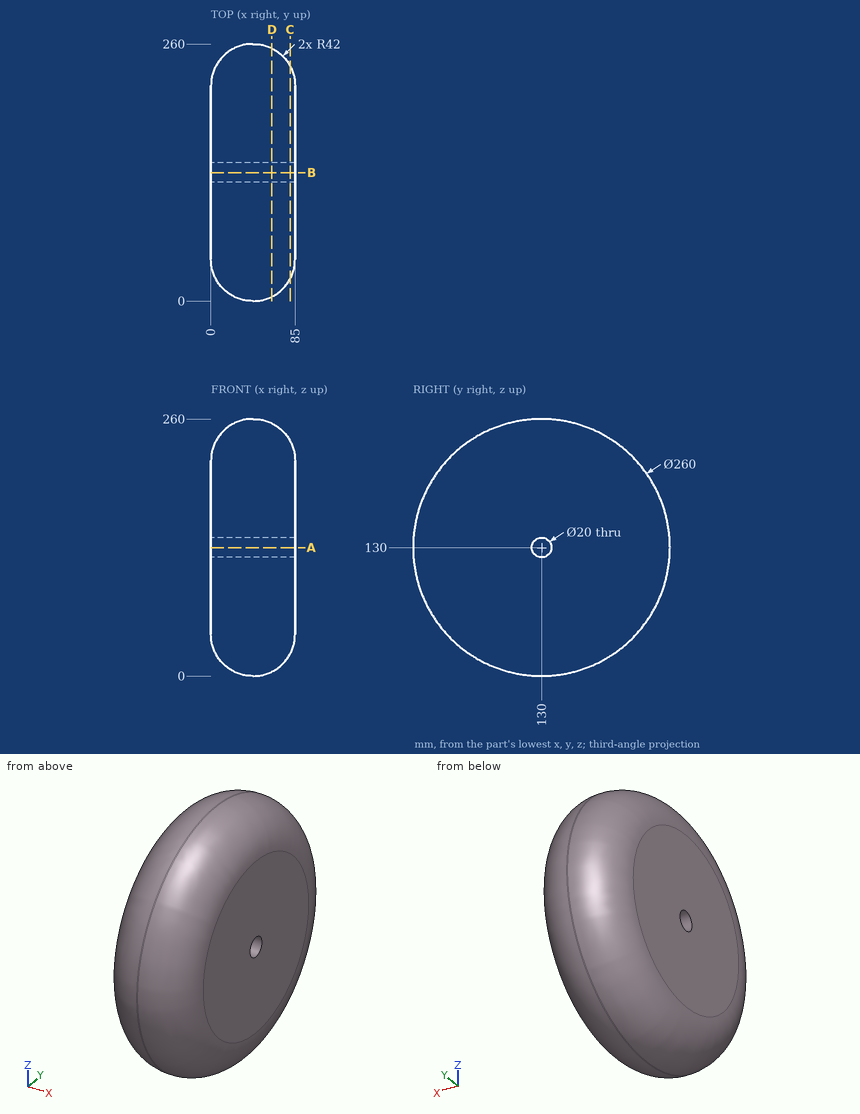
Drawing for the job (mm, zero at the part's lowest x, y, z). Round coordinates to 2 decimals unless told otherwise and drop trailing zeros. Order: outer loops, then holes, each group sorted by start corner. A loop starts at its lowest first (then second) coordinate and runs counter-clockwise, first axis right, second up.
Item 1: Pin check, flat tips, straight feed: pin 1 (8 mm diameter, centred on y = 37.5, z = 58, fed in from +X); pin 2 (5 mm diameter, centred on x = 32, z = 65, fed in from +Y); pin 3 (1.5 mm diameter, centred on x = 33, y = 86, fed in from -Z). Stop position of each tip, or through.
Item 2: Saw through at C-C on x = 80. Write the cut outline in (y, z), then the cut area to 3 significant figures.
Item 3: Probe line 1 along Z through (x, y) = (20, 130); line 2 along Z through (x, y) = (66, 130); line 3 along Z through (x, y) = (66.5, 27). List the from-to ranges inside material, lowest first.
Item 4: Saw through at A-A on z = 130. Write the cut outline in (x, y), then the cut area to 3 significant figures.
Item 5: Saw through at D-D on x = 61.5. Write the cut outline in (y, z).
Reported:
1. pin 1: stops at x = 76.59
1. pin 2: stops at y = 242.76
1. pin 3: stops at z = 8.39
2. outline: circle Ø215.75 at (130, 130); hole circle Ø20 at (130, 130)
2. area: 36,200 mm2
3. line 1: z = 6.22 to 120, 140 to 253.78
3. line 2: z = 6.86 to 120, 140 to 253.14
3. line 3: z = 63.12 to 196.88
4. outline: (0, 42) arc R42 ccw to (42, 0) - (43, 0) arc R42 ccw to (85, 42) - (85, 120) - (0, 120) - close; (0, 140) - (85, 140) - (85, 218) arc R42 ccw to (43, 260) - (42, 260) arc R42 ccw to (0, 218) - close
4. area: 18,900 mm2
5. outline: circle Ø251.41 at (130, 130); hole circle Ø20 at (130, 130)
